Model file for the job. Use its own axes, mm. A direction names the side the tool comes from. Round coordinates to 2 decimals unless told otherwise and drop trailing zeros. Order: outer loops, then holes, each group sorted by start corner. A loop starts at its lowest first (then second) coordinate and runs counter-clockwise, first axis right, second up. Notation, with made-up numbers: (49, -14) - (70, -14) arc R15 ccw to (70, -4) - close; hole circle Ø11 at (5, 81). An arc over 180 degrees is marked (long way). Answer as CSV lines item,"result". Start each with the question number.
1. Band-saw the part on B-B on y = -4.7. List the corners of the cut face in (x, z).
2. Pull direction Y, two halves, no side cores. Call faces 1 (the face through (-2, -1.905, 17)), 2 (the face through (6.835, -0.939, 16.91)), 3 (the face through (16, -5.715, 16)): released by +Y, released by -Y, zero draft, split by the parting line, or undercut.
3. Pin check, flat tip, straight feed: pin 1 Ø0.6 at (x, y) = (17, -4.5) entering from +Z. Stop position of the tip, or through.
4. Band-saw the part on C-C on z = 17.5. State how many separate pieces and enclosed holes the cut face has, then the cut area to 3 significant figures.
5. 3-axis set-ups, long thin cutter, end or side, ignore diameter. For faces 4 (the face through (0.74, -0.94, 16.91)), 5 (the face through (5, -1.905, 17)), 6 (the face through (32, -1, 17.974)), 7 (the face through (32.87, -0.94, 16.88)): which of +Z, -Z, +X, -X, +Y, -Y reach the whole face in a straight line?
6. Band-saw the part on A-A on x = 3. List the corners of the cut face in (y, z) (3 decimals), then the cut area to 3 significant figures.
7. Wall check: line 1 along Z through (x, y) = (9.5, -3.55); line 2 along Z through (x, y) = (15.5, -4.65); line 3 along Y through (x, z) = (28.5, 17.5) (3 decimals). Give the ranges that are in metal, low to high. Write a range as [from, to].
```python
from build123d import *

# Parameters (mm, degrees)
F1_DEPTH = 3.81
F4_DEPTH = 71.628
F5_SCALE = 0.5


with BuildPart() as f1:
    # F0 (on Front) → F1 (new body)
    with BuildSketch(Plane.XZ):
        Polygon((-38.4448663006, 16.8945933835), (-38.4448663006, 14.7355933835), (33.1831336994, 14.7355933835), (33.1831336994, 16.8945933835), (28.6111336994, 16.8945933835), (27.0871336994, 16.8945933835), (22.5151336994, 16.8945933835), (20.9911336994, 16.8945933835), (16.4191336994, 16.8945933835), (14.8951336994, 16.8945933835), (10.3231336994, 16.8945933835), (8.7991336994, 16.8945933835), (4.2271336994, 16.8945933835), (2.7031336994, 16.8945933835), (-1.8688663006, 16.8945933835), (-3.3928663006, 16.8945933835), (-7.9648663006, 16.8945933835), (-9.4888663006, 16.8945933835), (-14.0608663006, 16.8945933835), (-15.5848663006, 16.8945933835), (-20.1568663006, 16.8945933835), (-21.6808663006, 16.8945933835), (-26.2528663006, 16.8945933835), (-27.7768663006, 16.8945933835), (-32.3488663006, 16.8945933835), (-33.8728663006, 16.8945933835), align=None)
        Polygon((-37.1748663006, 21.2125933835), (-38.4448663006, 16.8945933835), (-33.8728663006, 16.8945933835), (-35.1428663006, 21.2125933835), align=None)
        Polygon((28.6111336994, 16.8945933835), (33.1831336994, 16.8945933835), (31.9131336994, 21.2125933835), (29.8811336994, 21.2125933835), align=None)
        Polygon((-31.0788663006, 21.2125933835), (-32.3488663006, 16.8945933835), (-27.7768663006, 16.8945933835), (-29.0468663006, 21.2125933835), align=None)
        Polygon((22.5151336994, 16.8945933835), (27.0871336994, 16.8945933835), (25.8171336994, 21.2125933835), (23.7851336994, 21.2125933835), align=None)
        Polygon((-24.9828663006, 21.2125933835), (-26.2528663006, 16.8945933835), (-21.6808663006, 16.8945933835), (-22.9508663006, 21.2125933835), align=None)
        Polygon((16.4191336994, 16.8945933835), (20.9911336994, 16.8945933835), (19.7211336994, 21.2125933835), (17.6891336994, 21.2125933835), align=None)
        Polygon((-18.8868663006, 21.2125933835), (-20.1568663006, 16.8945933835), (-15.5848663006, 16.8945933835), (-16.8548663006, 21.2125933835), align=None)
        Polygon((10.3231336994, 16.8945933835), (14.8951336994, 16.8945933835), (13.6251336994, 21.2125933835), (11.5931336994, 21.2125933835), align=None)
        Polygon((-12.7908663006, 21.2125933835), (-14.0608663006, 16.8945933835), (-9.4888663006, 16.8945933835), (-10.7588663006, 21.2125933835), align=None)
        Polygon((4.2271336994, 16.8945933835), (8.7991336994, 16.8945933835), (7.5291336994, 21.2125933835), (5.4971336994, 21.2125933835), align=None)
        Polygon((-6.6948663006, 21.2125933835), (-7.9648663006, 16.8945933835), (-3.3928663006, 16.8945933835), (-4.6628663006, 21.2125933835), align=None)
        Polygon((-1.8688663006, 16.8945933835), (2.7031336994, 16.8945933835), (1.4331336994, 21.2125933835), (-0.5988663006, 21.2125933835), align=None)
    extrude(amount=F1_DEPTH)

    # F3 (on plane+point) → F4 (join, through all)
    with BuildSketch(Plane.YZ.offset(33.1831336994)):
        Polygon((-11.43, 14.7355933835), (-3.81, 14.7355933835), (-3.81, 16.8945933835), (-7.62, 16.8945933835), (-7.62, 19.0535933835), (-11.43, 19.0535933835), (-11.43, 16.8945933835), align=None)
    extrude(amount=-F4_DEPTH)


with BuildPart() as f1_1:
    # F5: moved
    add(f1.part.scale(F5_SCALE).moved(Location((16.5915668497, 0, 7.3677966917))))


solid = f1_1.part
```
Reply:
1,outline,"(-2.63, 14.74) - (33.18, 14.74) - (33.18, 16.89) - (-2.63, 16.89) - close"
2,face 1,"undercut"
2,face 2,"zero draft"
2,face 3,"released by -Y"
3,pin 1,"stops at z = 16.89"
4,separate pieces,"12"
4,enclosed holes,"0"
4,area,"29.6 mm2"
5,face 4,"+Z, +Y"
5,face 5,"+Z, +X, -X"
5,face 6,"+Z, +X, -X, +Y, -Y"
5,face 7,"+Z, +X, +Y"
6,outline,"(-5.715, 14.736) - (0, 14.736) - (0, 15.815) - (-3.81, 15.815) - (-3.81, 16.895) - (-5.715, 16.895) - close"
6,area,"8.23 mm2"
7,line 1,"z = [14.74, 15.82]"
7,line 2,"z = [14.74, 16.89]"
7,line 3,"y = [-1.905, 0]"
